Design review of the part built by this model. Coordinates are the model's own, in mm. A direction names the side the tool comes from. Give positions to 0.01 mm unless a question says otherwise; leave off trailing zeros. Write each loop counter-clockwise with the first axis right and the second up, starting at its lowest first coordinate (ties: lowest second). Pieces come first, ordered by that corner, then holes.
```python
from build123d import *

# Parameters (mm, degrees)
F0_W     = 7
F0_H     = 7
F1_DEPTH = 7
F2_DEPTH = 11
F3_DEPTH = 2


with BuildPart() as f1:
    # F0 (on Top) → F1 (new body)
    with BuildSketch(Plane.XY):
        with Locations((22.4848273695, -11.8474444523)):
            Rectangle(F0_W, F0_H)
    extrude(amount=F1_DEPTH)



with BuildPart() as f2:
    # F0 (on Top) → F2 (new body)
    with BuildSketch(Plane.XY):
        with BuildLine():
            Line((34.9848273695, -3.1174444523), (34.9848273695, -2.1174444523))
            ThreePointArc((34.9848273695, -2.1174444523), (32.4848273695, -4.6174444523), (34.9848273695, -7.1174444523))
            Line((34.9848273695, -7.1174444523), (34.9848273695, -6.1174444523))
            ThreePointArc((34.9848273695, -6.1174444523), (33.4848273695, -4.6174444523), (34.9848273695, -3.1174444523))
        make_face()
        with BuildLine():
            Line((34.9848273695, -3.3474444523), (34.9848273695, -3.1174444523))
            ThreePointArc((34.9848273695, -3.1174444523), (33.4848273695, -4.6174444523), (34.9848273695, -6.1174444523))
            Line((34.9848273695, -6.1174444523), (34.9848273695, -5.8874444523))
            Line((34.9848273695, -5.8874444523), (34.9848273695, -3.3474444523))
        make_face()
        with BuildLine():
            ThreePointArc((36.4848273695, -4.6174444523), (36.0454875412, -3.5567842806), (34.9848273695, -3.1174444523))
            Line((34.9848273695, -3.1174444523), (34.9848273695, -3.3474444523))
            Line((34.9848273695, -3.3474444523), (34.9848273695, -5.8874444523))
            Line((34.9848273695, -5.8874444523), (34.9848273695, -6.1174444523))
            ThreePointArc((34.9848273695, -6.1174444523), (36.0454875412, -5.6781046241), (36.4848273695, -4.6174444523))
        make_face()
        with BuildLine():
            ThreePointArc((36.9848273695, -3.1174444523), (36.1028613582, -2.3813764748), (34.9848273695, -2.1174444523))
            Line((34.9848273695, -2.1174444523), (34.9848273695, -3.1174444523))
            ThreePointArc((34.9848273695, -3.1174444523), (36.0454875412, -3.5567842806), (36.4848273695, -4.6174444523))
            ThreePointArc((36.4848273695, -4.6174444523), (36.0454875412, -5.6781046241), (34.9848273695, -6.1174444523))
            Line((34.9848273695, -6.1174444523), (34.9848273695, -7.1174444523))
            ThreePointArc((34.9848273695, -7.1174444523), (36.1028613582, -6.8535124298), (36.9848273695, -6.1174444523))
            Line((36.9848273695, -6.1174444523), (36.9848273695, -3.1174444523))
        make_face()
        with BuildLine():
            ThreePointArc((37.4848273695, -4.6174444523), (37.3565356146, -3.8268750373), (36.9848273695, -3.1174444523))
            Line((36.9848273695, -3.1174444523), (36.9848273695, -6.1174444523))
            ThreePointArc((36.9848273695, -6.1174444523), (37.3565356146, -5.4080138674), (37.4848273695, -4.6174444523))
        make_face()
    extrude(amount=F2_DEPTH)


with BuildPart() as f2b:
    # F0 (on Top) → F2, piece 2 (new body)
    with BuildSketch(Plane.XY):
        with BuildLine():
            ThreePointArc((36.4848273695, -12.0774444523), (36.0454875412, -11.0167842806), (34.9848273695, -10.5774444523))
            Line((34.9848273695, -10.5774444523), (34.9848273695, -10.8074444523))
            Line((34.9848273695, -10.8074444523), (34.9848273695, -13.3474444523))
            Line((34.9848273695, -13.3474444523), (34.9848273695, -13.5774444523))
            ThreePointArc((34.9848273695, -13.5774444523), (36.0454875412, -13.1381046241), (36.4848273695, -12.0774444523))
        make_face()
        with BuildLine():
            ThreePointArc((37.4848273695, -12.0774444523), (37.3565356146, -11.2868750373), (36.9848273695, -10.5774444523))
            Line((36.9848273695, -10.5774444523), (36.9848273695, -13.5774444523))
            ThreePointArc((36.9848273695, -13.5774444523), (37.3565356146, -12.8680138674), (37.4848273695, -12.0774444523))
        make_face()
        with BuildLine():
            ThreePointArc((36.9848273695, -10.5774444523), (36.1028613582, -9.8413764748), (34.9848273695, -9.5774444523))
            Line((34.9848273695, -9.5774444523), (34.9848273695, -10.5774444523))
            ThreePointArc((34.9848273695, -10.5774444523), (36.0454875412, -11.0167842806), (36.4848273695, -12.0774444523))
            ThreePointArc((36.4848273695, -12.0774444523), (36.0454875412, -13.1381046241), (34.9848273695, -13.5774444523))
            Line((34.9848273695, -13.5774444523), (34.9848273695, -14.5774444523))
            ThreePointArc((34.9848273695, -14.5774444523), (36.1028613582, -14.3135124298), (36.9848273695, -13.5774444523))
            Line((36.9848273695, -13.5774444523), (36.9848273695, -10.5774444523))
        make_face()
        with BuildLine():
            Line((34.9848273695, -10.8074444523), (34.9848273695, -10.5774444523))
            ThreePointArc((34.9848273695, -10.5774444523), (33.4848273695, -12.0774444523), (34.9848273695, -13.5774444523))
            Line((34.9848273695, -13.5774444523), (34.9848273695, -13.3474444523))
            Line((34.9848273695, -13.3474444523), (34.9848273695, -10.8074444523))
        make_face()
        with BuildLine():
            Line((34.9848273695, -10.5774444523), (34.9848273695, -9.5774444523))
            ThreePointArc((34.9848273695, -9.5774444523), (32.4848273695, -12.0774444523), (34.9848273695, -14.5774444523))
            Line((34.9848273695, -14.5774444523), (34.9848273695, -13.5774444523))
            ThreePointArc((34.9848273695, -13.5774444523), (33.4848273695, -12.0774444523), (34.9848273695, -10.5774444523))
        make_face()
    extrude(amount=F2_DEPTH)


with BuildPart() as f1_1:
    add(f1.part)

    add(f2.part)  # F3 merges F2

    add(f2b.part)  # F3 merges F2b
    # F0 (on Top) → F3 (join)
    with BuildSketch(Plane.XY):
        with BuildLine():
            Line((34.9848273695, -1.3474444523), (5.9848273695, -1.3474444523))
            Line((5.9848273695, -1.3474444523), (5.9848273695, -15.3474444523))
            Line((5.9848273695, -15.3474444523), (18.9848273695, -15.3474444523))
            Line((18.9848273695, -15.3474444523), (18.9848273695, -8.3474444523))
            Line((18.9848273695, -8.3474444523), (25.9848273695, -8.3474444523))
            Line((25.9848273695, -8.3474444523), (25.9848273695, -15.3474444523))
            Line((25.9848273695, -15.3474444523), (34.9848273695, -15.3474444523))
            Line((34.9848273695, -15.3474444523), (34.9848273695, -14.5774444523))
            ThreePointArc((34.9848273695, -14.5774444523), (32.4848273695, -12.0774444523), (34.9848273695, -9.5774444523))
            Line((34.9848273695, -9.5774444523), (34.9848273695, -7.1174444523))
            ThreePointArc((34.9848273695, -7.1174444523), (32.4848273695, -4.6174444523), (34.9848273695, -2.1174444523))
            Line((34.9848273695, -2.1174444523), (34.9848273695, -1.3474444523))
        make_face()
        with BuildLine():
            Line((34.9848273695, -14.5774444523), (34.9848273695, -15.3474444523))
            Line((34.9848273695, -15.3474444523), (36.9848273695, -15.3474444523))
            Line((36.9848273695, -15.3474444523), (36.9848273695, -13.5774444523))
            ThreePointArc((36.9848273695, -13.5774444523), (36.1028613582, -14.3135124298), (34.9848273695, -14.5774444523))
        make_face()
        with BuildLine():
            ThreePointArc((36.9848273695, -6.1174444523), (36.1028613582, -6.8535124298), (34.9848273695, -7.1174444523))
            Line((34.9848273695, -7.1174444523), (34.9848273695, -9.5774444523))
            ThreePointArc((34.9848273695, -9.5774444523), (36.1028613582, -9.8413764748), (36.9848273695, -10.5774444523))
            Line((36.9848273695, -10.5774444523), (36.9848273695, -6.1174444523))
        make_face()
        with BuildLine():
            Line((36.9848273695, -1.3474444523), (34.9848273695, -1.3474444523))
            Line((34.9848273695, -1.3474444523), (34.9848273695, -2.1174444523))
            ThreePointArc((34.9848273695, -2.1174444523), (36.1028613582, -2.3813764748), (36.9848273695, -3.1174444523))
            Line((36.9848273695, -3.1174444523), (36.9848273695, -1.3474444523))
        make_face()
    extrude(amount=F3_DEPTH)


solid = f1_1.part
```
(1) Consider section B-B, the plane z = 9. Give the boundary of the cut face in (x, y).
Resolved:
outline: circle Ø5 at (34.98, -12.08); circle Ø5 at (34.98, -4.62)
(2) To check wall thickness, follow L1, parallel to X at y = -9.25, z = 4.25; L2, parallel to Z at x = 26, y = -6.5; L3, parallel to Y at x = 25.5, z = 6. State the ranges of each line that lie inside material, in increasing order.
Resolved:
L1: x = 18.98 to 25.98
L2: z = 0 to 2
L3: y = -15.35 to -8.35
(3) Consider section C-C, the plane y = -9.25. Give the boundary of the cut face in (x, z), then the cut area to 3 significant figures.
Resolved:
outline: (5.98, 0) - (36.98, 0) - (36.98, 2) - (25.98, 2) - (25.98, 7) - (18.98, 7) - (18.98, 2) - (5.98, 2) - close
area: 97.0 mm2
(4) Mouldability with a two-part tool opening along Y and no side actions: class faces 4 (the face through (36.985, -8, 1)), 5 (the face through (22, -8.347, 4)), 6 (the face through (36.985, -14, 1)) as pulls with the +Y half, pulls with the -Y half, needs draft (parallel to the pull), parting line crosses it, or undercut.
Resolved:
face 4: undercut
face 5: pulls with the +Y half
face 6: needs draft
(5) Consider section D-D, the plane x = 21. Give the boundary of the cut face in (y, z).
Resolved:
outline: (-15.35, 0) - (-1.35, 0) - (-1.35, 2) - (-8.35, 2) - (-8.35, 7) - (-15.35, 7) - close
(6) Tool access review of faces 1 (the face through (25.985, -12, 4)), 2 (the face through (36.985, -2, 1)), 3 (the face through (22, -12, 7)): name each direction out of +Z, -Z, +X, -X, +Y, -Y from which nothing blocks a thin tool from reaching the whole face with its end or side.
Resolved:
face 1: +Z, +Y, -Y
face 2: +Z, -Z, +X, +Y
face 3: +Z, -X, +Y, -Y
(7) Consider section A-A, the plane z = 2.75. Give the boundary of the cut face in (x, y), then the cut area to 3 significant figures.
Resolved:
outline: (18.98, -15.35) - (25.98, -15.35) - (25.98, -8.35) - (18.98, -8.35) - close; circle Ø5 at (34.98, -12.08); circle Ø5 at (34.98, -4.62)
area: 88.3 mm2
(8) Clearance check with flat-ended pins moving along their axes: P1, Ø2, axis at x = 12.5, y = -5.5, coming from the +Z side; P2, Ø1.4, axis at y = -15, z = 1, coming from the +X side; P3, Ø4, axis at y = -13, z = 4.5, coming from the -X side; P4, Ø4, axis at x = 10, z = 5, coming from the +Y side. State where each tip first meets the part, or that it passes through.
Resolved:
P1: stops at z = 2
P2: stops at x = 36.98
P3: stops at x = 18.98
P4: passes through
